```python
from build123d import *

# Parameters (mm, degrees)
SKETCH1_W           = 105
SKETCH1_H           = 50
BOSS_EXTRUDE1_DEPTH = 15
SKETCH4_R           = 8
BOSS_EXTRUDE2_DEPTH = 8
SKETCH5_R           = 25
BOSS_EXTRUDE3_DEPTH = 20


with BuildPart() as part:
    # Sketch1 → Boss-Extrude1 (new body)
    with BuildSketch(Plane.XY):
        Rectangle(SKETCH1_W, SKETCH1_H)
    extrude(amount=BOSS_EXTRUDE1_DEPTH)

    # Sketch4 → Boss-Extrude2 (add)
    with BuildSketch(Plane.ZY.offset(52.5)):
        with BuildLine():
            Line((0, -25), (0, 25))
            Line((0, 25), (-20, 22.870754113))
            ThreePointArc((-20, 22.870754113), (-40.565127043, 0), (-20, -22.870754113))
            Line((-20, -22.870754113), (0, -25))
        make_face()
        with Locations(Location((-20, 0, 0), (0, 0, 270))):
            Circle(SKETCH4_R, mode=Mode.SUBTRACT)
    boss_extrude2 = extrude(amount=-BOSS_EXTRUDE2_DEPTH)

    # Mirror1: Boss-Extrude2 across plane
    add(boss_extrude2.mirror(Plane(origin=(0, 0, 0), x_dir=(0, 0, 1), z_dir=(1, 0, 0))))

    # Sketch5 → Boss-Extrude3 (add)
    with BuildSketch(Plane.XY.offset(15)):
        with Locations(Location((0, 0, 0), (0, 0, 270))):
            Circle(SKETCH5_R)
        with BuildLine():
            Line((3, 12.1346611), (3, 15.1346611))
            Line((3, 15.1346611), (-3, 15.1346611))
            Line((-3, 15.1346611), (-3, 12.1346611))
            ThreePointArc((-3, 12.1346611), (0, -12.5), (3, 12.1346611))
        make_face(mode=Mode.SUBTRACT)
    extrude(amount=BOSS_EXTRUDE3_DEPTH)


solid = part.part
```
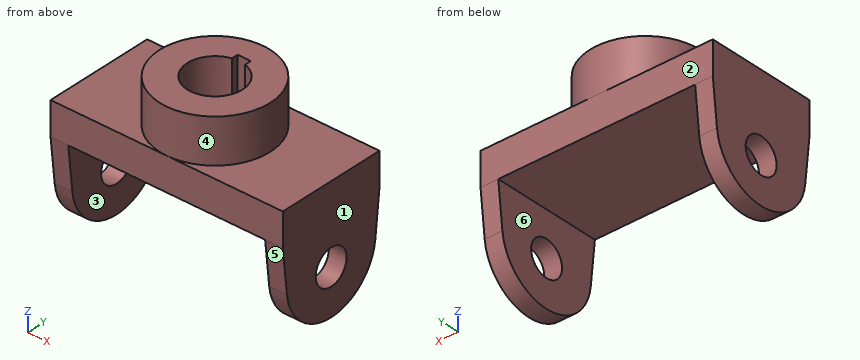
Geometry: final body of the model. Coordinates: model frame, mm. Face numbers are marked on the shaded views. A direction names the side the tool comes from. Round coordinates to 2 decimals unless told otherwise and drop trailing zeros. Order: outer loops, then holes, each group sorted by start corner. A loop starts at its lowest first (then second) coordinate and runs counter-clockwise, first axis right, second up. Notation, with made-up numbers: (-19, -5) -> (27, -5) arc R34 ccw to (27, 30) -> close; hole circle Ø6 at (-4.5, 21.5). An arc over 180 degrees is marked (long way). Use one line per item in the form item = value. Start each with the question number.
1. Cut plane D-D (y = 0). Return the cut outline in (x, z), then the cut area to 3 significant figures.
2. Cut plane B-B (x = 7). Return the cut outline in (y, z).
3. Cut plane A-A (y = 6). Return the cut outline in (x, z), then the cut area to 3 significant figures.
4. Reachability of the marked faces 4, 5 and 6 from +Z, -Z, +X, -X, +Y, -Y: full face, straight path, thin tool, end or side. Return the list, or none.
5. Pin query (flat end, axial travel): pin 1 Ø1.5 at (x, z) = (-24.5, -1) entering from +Y; pin 2 Ø1.5 at (y, z) = (14, 27.5) entering from +X; pin 3 Ø6 at (y, z) = (-8.5, 23.5) entering from +X; pin 4 Ø2 at (x, y) = (31.5, -9) entering from +Z. Return the tip coordinate at first contact, or that it passes through.
6. Line query: probe 1 along X at (y, z) = (-20, -20); probe 2 along X at (y, z) = (0, 23); probe 3 along Z at (x, y) = (-10, 14.5). Output: solid intervals per line, ascending.
7. Draft query along X for the marked faces 1, 2 and 3. Return one class per face: pulls with the +X half, pulls with the -X half, needs draft (parallel to the pull), parting line crosses it, or undercut.
8. Cut plane C-C (z = 20.5). Return the cut outline in (x, y), then the cut area to 3 significant figures.
Solution:
q1.outline = (-52.5, -40.57) -> (-44.5, -40.57) -> (-44.5, -28) -> (-52.5, -28) -> close; (-52.5, -12) -> (-44.5, -12) -> (-44.5, 0) -> (44.5, 0) -> (44.5, -12) -> (52.5, -12) -> (52.5, 15) -> (25, 15) -> (25, 35) -> (12.5, 35) -> (12.5, 15) -> (-12.5, 15) -> (-12.5, 35) -> (-25, 35) -> (-25, 15) -> (-52.5, 15) -> close; (44.5, -40.57) -> (52.5, -40.57) -> (52.5, -28) -> (44.5, -28) -> close
q1.area = 2,470 mm^2
q2.outline = (-25, 0) -> (25, 0) -> (25, 15) -> (24, 15) -> (24, 35) -> (10.36, 35) -> (10.36, 15) -> (-10.36, 15) -> (-10.36, 35) -> (-24, 35) -> (-24, 15) -> (-25, 15) -> close
q3.outline = (-52.5, -39.77) -> (-44.5, -39.77) -> (-44.5, -25.29) -> (-52.5, -25.29) -> close; (-52.5, -14.71) -> (-44.5, -14.71) -> (-44.5, 0) -> (44.5, 0) -> (44.5, -14.71) -> (52.5, -14.71) -> (52.5, 15) -> (24.27, 15) -> (24.27, 35) -> (10.97, 35) -> (10.97, 15) -> (-10.97, 15) -> (-10.97, 35) -> (-24.27, 35) -> (-24.27, 15) -> (-52.5, 15) -> close; (44.5, -39.77) -> (52.5, -39.77) -> (52.5, -25.29) -> (44.5, -25.29) -> close
q3.area = 2,570 mm^2
q4.face_4 = +Z
q4.face_5 = -Z, +X, -X, -Y
q4.face_6 = -Z, +Y, -Y
q5.pin_1 = through
q5.pin_2 = 21.2
q5.pin_3 = 24.39
q5.pin_4 = 15
q6.probe_1 = -52.5 to -44.5, 44.5 to 52.5
q6.probe_2 = -25 to -12.5, 12.5 to 25
q6.probe_3 = 0 to 35
q7.face_1 = pulls with the +X half
q7.face_2 = needs draft
q7.face_3 = undercut
q8.outline = circle Ø50 at (0, 0); hole (-3, 12.13) arc R12.5 ccw (long way) to (3, 12.13) -> (3, 15.13) -> (-3, 15.13) -> close
q8.area = 1,460 mm^2
